Verification items for the finished model (mm, model axes). A direction names the side the tool comes from. Give positions to 0.01 mm unless a question says otherwise; leave off trailing zeros. Order: outer loops, then holes, each group sorted by start corner. A loop starts at its lowest first (then second) coordinate and runs counter-clockwise, first axis right, second up.
(1) Sectioned sample at A-A on z = 29.5. Record the cut outline in (x, y).
(2) Gauge pin test, flat ends, axial feed: pin 1 (5.5 mm diameter, centred on x = -10.19, y = -11.6, fed in from +Z); pin 2 (1.6 mm diameter, centred on x = 25, y = -11, fed in from +Z); pin 3 (12 mm diameter, centred on y = 1, z = 29.5, fed in from +X). Record the tip position at first contact, or that the pin passes through.
(3) Scan lines: L1, parallel to Y at x = 16.5, z = 32; L2, parallel to Z at x = 22.5, y = 22.5; L3, parallel to Y at x = -3, z = 43. Record each from-to range of solid material in increasing order.
(4) Mould release check, pull along Z, two halves, no side actions. Record for faces 4 (the face through (23.56, 25.71, 4.52)), 5 (the face through (4.179, -9.938, 74.233)), 6 (the face through (-9, -10, 3)): pulls with the +Z half, pulls with the -Z half, needs draft (parallel to the pull), parting line crosses it, or undercut.
(5) Access from +Z, -Z, +X, -X, +Y, -Y to the whole of each face (thin tool, end or side, straight path). Record for faces 1 (the face through (4.663, -7.758, 39.952)), 2 (the face through (28.3, 12.9, 7)), 3 (the face through (-6, 16, 9)).
```python
from build123d import *

# Parameters (mm, degrees)
F0_W         = 45
F0_H         = 45
F0_R         = 1.7
F1_DEPTH     = 6
F2_R         = 1.7
F3_DEPTH     = 3
F4_R         = 4
F5_R         = 21.5
F6_DEPTH     = 3
F7_SIZE      = 1
F8_R         = 16.5
F9_DEPTH     = 65
F10_R        = 21.5
F11_DEPTH    = 4.8
F12_S5_R     = 16.5
F12_T6_DEPTH = 32
F13_R        = 14.5
F14_DEPTH    = 100


# Not quite as in the source:
# - a fillet or chamfer that OpenCascade refuses, or shapes differently, is made with other operations: its cross-section is extruded or revolved along the edge and cut away or added


with BuildPart() as f1:
    # F0 (on Top) → F1 (new body)
    with BuildSketch(Plane.XY):
        with Locations((7.8061202839, 6.3967237547)):
            Rectangle(F0_W, F0_H)
        with Locations((-10.1938797161, -11.6032762453)):
            Circle(F0_R, mode=Mode.SUBTRACT)
        with Locations((25.8061202839, -11.6032762453)):
            Circle(F0_R, mode=Mode.SUBTRACT)
        with Locations((-10.1938797161, 24.3967237547)):
            Circle(F0_R, mode=Mode.SUBTRACT)
        with Locations((25.8061202839, 24.3967237547)):
            Circle(F0_R, mode=Mode.SUBTRACT)
    extrude(amount=F1_DEPTH)

    # F2 (on face) → F3 (cut)
    with BuildSketch(Plane.XY.offset(6)):
        Polygon((-11.694990416, 21.7967237547), (-8.6927690162, 21.7967237547), (-7.1916583163, 24.3967237547), (-8.6927690162, 26.9967237547), (-11.694990416, 26.9967237547), (-13.1961011159, 24.3967237547), align=None)
        with Locations((-10.1938797161, 24.3967237547)):
            Circle(F2_R, mode=Mode.SUBTRACT)
        Polygon((24.305009584, 21.7967237547), (27.3072309838, 21.7967237547), (28.8083416837, 24.3967237547), (27.3072309838, 26.9967237547), (24.305009584, 26.9967237547), (22.8038988841, 24.3967237547), align=None)
        with Locations((25.8061202839, 24.3967237547)):
            Circle(F2_R, mode=Mode.SUBTRACT)
        Polygon((-8.6927690162, -9.0032762453), (-11.694990416, -9.0032762453), (-13.1961011159, -11.6032762453), (-11.694990416, -14.2032762453), (-8.6927690162, -14.2032762453), (-7.1916583163, -11.6032762453), align=None)
        with Locations((-10.1938797161, -11.6032762453)):
            Circle(F2_R, mode=Mode.SUBTRACT)
        Polygon((27.3072309838, -9.0032762453), (24.305009584, -9.0032762453), (22.8038988841, -11.6032762453), (24.305009584, -14.2032762453), (27.3072309838, -14.2032762453), (28.8083416837, -11.6032762453), align=None)
        with Locations((25.8061202839, -11.6032762453)):
            Circle(F2_R, mode=Mode.SUBTRACT)
    extrude(amount=-F3_DEPTH, mode=Mode.SUBTRACT)

    # F4
    f4_edges = [f1.edges().sort_by_distance(p)[0] for p in [
        (-14.69388, 28.896724, 3),
        (30.30612, 28.896724, 3),
        (30.30612, -16.103276, 3),
        (-14.69388, -16.103276, 3),
    ]]
    fillet(f4_edges, radius=F4_R)

    # F5 (on face) → F6 (join)
    with BuildSketch(Plane.XY.offset(6)):
        with Locations((7.8061202839, 6.3967237547)):
            Circle(F5_R)
    extrude(amount=F6_DEPTH)

    # F7
    f7_edges = [f1.edges().sort_by_distance(p)[0] for p in [
        (-13.69388, 6.396724, 9),
    ]]
    chamfer(f7_edges, length=F7_SIZE)

    # F8 (on face) → F9 (join)
    with BuildSketch(Plane.XY.offset(9)):
        with Locations((7.8061202839, 6.3967237547)):
            Circle(F8_R)
    extrude(amount=F9_DEPTH)

    # F10 (on face) → F11 (join)
    with BuildSketch(Plane.XY.offset(74)):
        with Locations((7.8061202839, 6.3967237547)):
            Circle(F10_R)
    extrude(amount=F11_DEPTH)

    # F12: chamfer of 5 on 1 edges, made by hand


with BuildPart() as f12_tool2:
    # F12_s3 → F12_t4 (revolve)
    with BuildSketch(Plane.XZ.offset(-6.3967237547)):
        Polygon((29.3061202839, 79), (24.3061202839, 74), (29.3061202839, 74), align=None)
    revolve(axis=Axis((7.8061202839, 6.3967237547, 74), (0, 0, 1)))

    # F12_s5 → F12_t6 (cut, symmetric)
    with BuildSketch(Plane.XY.offset(76.5)):
        with Locations((7.8061202839, 6.3967237547)):
            Circle(F12_S5_R)
    extrude(amount=F12_T6_DEPTH, both=True, mode=Mode.SUBTRACT)


with BuildPart() as f1_1:
    add(f1.part)

    # F12_t1: cut F12_tool2
    add(f12_tool2.part, mode=Mode.SUBTRACT)

    # F13 (on face) → F14 (cut)
    with BuildSketch(Plane.XY.offset(78.8)):
        with Locations((7.8061202839, 6.3967237547)):
            Circle(F13_R)
    extrude(amount=-F14_DEPTH, mode=Mode.SUBTRACT)


solid = f1_1.part
```
Ans:
1. outline: circle Ø33 at (7.81, 6.4); hole circle Ø29 at (7.81, 6.4)
2. pin 1: stops at z = 6
2. pin 2: stops at z = 3
2. pin 3: stops at x = 24.31
3. L1: y = -7.63 to -5.21, 18 to 20.42
3. L2: z = 0 to 6
3. L3: y = -6.07 to -3.27, 16.07 to 18.87
4. face 4: needs draft
4. face 5: undercut
4. face 6: pulls with the +Z half
5. face 1: +Z, -Z
5. face 2: +Z
5. face 3: none
